Geometry check sheet. Reference: drawing and pictorial views, mm from the part's lowest x, y, z. A direction names the side the tool comes from. Give positions to 0.01 mm unless a question says otherwise; leave off trailing zeros. Order: outer loops, then holes, each group sorted by start corner. A loop starts at its lowest first (then second) coordinate and runs counter-clockwise, first axis right, second up.
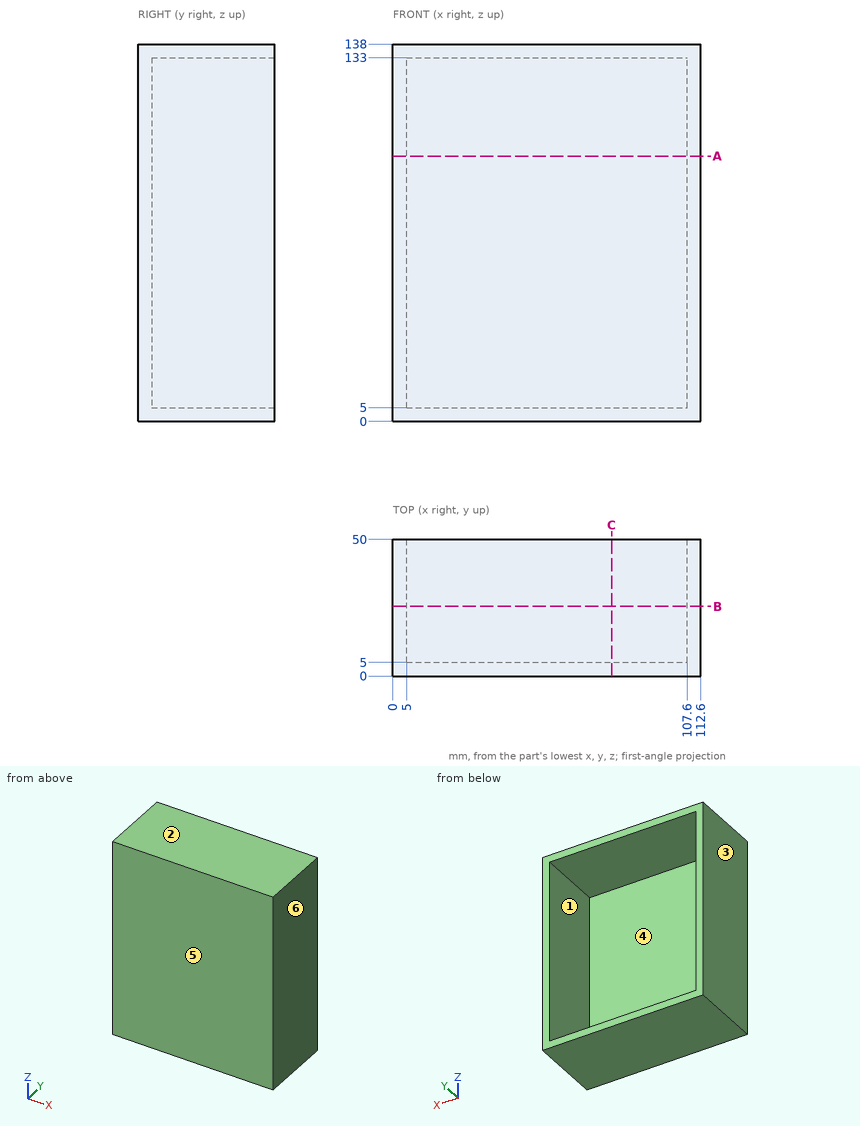
(1) Release check for a two-part mould opening along X. For the marked faces 3, 4, 5 and 6 record: released by +X, released by -X, zero draft, split by the parting line, or undercut.
Response values:
face 3: released by -X
face 4: undercut
face 5: zero draft
face 6: released by +X
(2) Cross-section at A-A on z = 97. Enter the section's corners in (x, y), then the cut area to 3 significant figures.
Response values:
outline: (0, 0) - (112.6, 0) - (112.6, 50) - (107.6, 50) - (107.6, 5) - (5, 5) - (5, 50) - (0, 50) - close
area: 1,010 mm2
(3) Cross-section at C-C on x = 80. Enter the section's corners in (y, z), then the cut area to 3 significant figures.
Response values:
outline: (0, 0) - (50, 0) - (50, 5) - (5, 5) - (5, 133) - (50, 133) - (50, 138) - (0, 138) - close
area: 1,140 mm2
(4) Set-up check for the marked faces 1 and 2: record each of +Z, -Z, +X, -X, +Y, -Y from which the full face is reachable in a straight line by a thin tool's end or side.
Response values:
face 1: +Y
face 2: +Z, +X, -X, +Y, -Y
(5) Gauge pin test, flat ends, axial feed: pin 1 Ø5 at (x, z) = (56, 18.5) entering from -Y; pin 2 Ø4 at (x, z) = (27.5, 92.5) entering from +Y. Record the tip position at first contact, or that the pin passes through.
Response values:
pin 1: stops at y = 0
pin 2: stops at y = 5
(6) Material ranges on L1, parallel to Z at x = 82, y = 5.5; L2, parallel to X at y = 33, z = 122; L3, parallel to Y at x = 107.5, z = 83.5, recorded low to high.
Response values:
L1: z = 0 to 5, 133 to 138
L2: x = 0 to 5, 107.6 to 112.6
L3: y = 0 to 5
(7) Cross-section at B-B on y = 25.5. Enter the section's corners in (x, z), then the cut area to 3 significant figures.
Response values:
outline: (0, 0) - (112.6, 0) - (112.6, 138) - (0, 138) - close; hole (5, 5) - (107.6, 5) - (107.6, 133) - (5, 133) - close
area: 2,410 mm2
